Build history of the part. All positions in model axes, mm. A direction names the side the tool comes from. Give positions to 0.01 mm unless a question says otherwise; leave off trailing zeros. Loops run counter-clockwise (first coordinate to the right, second up) from the corner with the lowest first, then second, coordinate; pieces in that order, holes last. Notation, with made-up numbers: (48.25, 15) -> (92.25, 15) arc R24 cw to (92.25, 34) -> close; hole circle Ø2 at (6.5, -1). An arc over 180 degrees is marked (long way). Answer in a Markdown table with one row per item. Add a question column.
from build123d import *

# Parameters (mm, degrees)
SKETCH1_R              = 8
BOSS_EXTRUDE1_DEPTH    = 130
FILLET1_R              = 20
SKETCH2_W              = 2
SKETCH2_H              = 130
BOSS_EXTRUDE4_DEPTH    = 30
CUT_EXTRUDE1_DEPTH     = 9
FILLET2_R              = 1
FILLET3_R              = 2
CUT_EXTRUDE2_START     = -11
CUT_EXTRUDE2_OUTLINE_W = 137
CUT_EXTRUDE2_OUTLINE_H = 54
CUT_EXTRUDE2_DEPTH     = 11
CUT_EXTRUDE3_DEPTH     = 50
SKETCH6_W              = 87.560859394
SKETCH6_H              = 110.580871242
SKETCH6_RX             = 28
SKETCH6_RY             = 6.639736886
SKETCH6_RY_2           = 5.950557319
BOSS_EXTRUDE7_DEPTH    = 1.5
SKETCH7_W              = 87.560859394
SKETCH7_H              = 1.5
CUT_EXTRUDE4_DEPTH     = 0.290435621
SKETCH8_W              = 87.560859394
SKETCH8_H              = 1.5
CUT_EXTRUDE5_DEPTH     = 0.290435621
SKETCH9_R              = 113.429913181
CUT_EXTRUDE6_DEPTH     = 135
SKETCH10_W             = 60.632055489
SKETCH10_H             = 78.176650268
BOSS_EXTRUDE8_DEPTH    = 4.5
SKETCH11_R             = 8.1
CUT_EXTRUDE7_DEPTH     = 135
SKETCH12_W             = 3
SKETCH12_H             = 110
BOSS_EXTRUDE9_DEPTH    = 51
FILLET4_R              = 10
FILLET5_R              = 1.5
FILLET7_R              = 1


# Read off the part's stored shape, not the designer's step: Cut-Extrude2
with BuildPart() as part:
    # Sketch1 → Boss-Extrude1 (new body)
    with BuildSketch(Plane(origin=(0, 0, 0), x_dir=(1, 0, 0), z_dir=(0, 1, 0))):
        with BuildLine():
            ThreePointArc((-62.734857267, 11), (-66.796876469, -10.22252415), (-55.185022832, 8))
            Line((-55.185022832, 8), (41.715308298, 8))
            ThreePointArc((41.715308298, 8), (53.327161935, -10.22252415), (49.265142733, 11))
            Line((49.265142733, 11), (-62.734857267, 11))
        make_face()
        with Locations(Location((-62.734857267, 0, 0), (0, 0, 270))):
            Circle(SKETCH1_R, mode=Mode.SUBTRACT)
        with Locations(Location((49.265142733, 0, 0), (0, 0, 270))):
            Circle(SKETCH1_R, mode=Mode.SUBTRACT)
    extrude(amount=BOSS_EXTRUDE1_DEPTH)

    # Fillet1
    fillet1_edges = [part.edges().sort_by_distance(p)[0] for p in [
        (41.715308298, 65, -8),
        (-55.185022832, 65, -8),
    ]]
    fillet(fillet1_edges, radius=FILLET1_R)

    # Sketch2 → Boss-Extrude4 (add)
    with BuildSketch(Plane(origin=(0, 0, -11), x_dir=(-1, 0, 0), z_dir=(0, 0, -1))):
        with Locations((7.734857267, 65)):
            Rectangle(SKETCH2_W, SKETCH2_H)
        with Locations((5.734857267, 65)):
            Rectangle(SKETCH2_W, SKETCH2_H)
    extrude(amount=BOSS_EXTRUDE4_DEPTH)

    # Sketch3 → Cut-Extrude1 (cut)
    with BuildSketch(Plane(origin=(0, 130, 0), x_dir=(1, 0, 0), z_dir=(0, 1, 0))):
        with BuildLine():
            Line((-34.151645411, 8), (20.681930877, 8))
            ThreePointArc((20.681930877, 8), (31.753545265, 4.655910508), (39.12271272, -4.258064516))
            ThreePointArc((39.12271272, -4.258064516), (58.425893512, -6.089387914), (49.265142733, 11))
            Line((49.265142733, 11), (-4.734857267, 11))
            Line((-4.734857267, 11), (-4.734857267, 41))
            Line((-4.734857267, 41), (-8.734857267, 41))
            Line((-8.734857267, 41), (-8.734857267, 11))
            Line((-8.734857267, 11), (-62.734857267, 11))
            ThreePointArc((-62.734857267, 11), (-71.895608046, -6.089387914), (-52.592427254, -4.258064516))
            ThreePointArc((-52.592427254, -4.258064516), (-45.223259799, 4.655910508), (-34.151645411, 8))
        make_face()
    extrude(amount=-CUT_EXTRUDE1_DEPTH, mode=Mode.SUBTRACT)

    # Fillet2
    fillet2_edges = [part.edges().sort_by_distance(p)[0] for p in [
        (-8.734857267, 60.5, -11),
        (-4.734857267, 60.5, -11),
    ]]
    fillet(fillet2_edges, radius=FILLET2_R)

    # Fillet3
    fillet3_edges = [part.edges().sort_by_distance(p)[0] for p in [
        (-4.734857267, 60.5, -41),
        (-8.734857267, 60.5, -41),
    ]]
    fillet(fillet3_edges, radius=FILLET3_R - 0.0001)  # a hair under: the kernel refuses the full size

    # Cut-Extrude2 outline → Cut-Extrude2 (cut)
    with BuildSketch(Plane.XZ.offset(CUT_EXTRUDE2_START)):
        with Locations((-6.5, -15)):
            Rectangle(CUT_EXTRUDE2_OUTLINE_W, CUT_EXTRUDE2_OUTLINE_H)
    extrude(amount=CUT_EXTRUDE2_DEPTH, mode=Mode.SUBTRACT)

    # Sketch5 → Cut-Extrude3 (cut)
    with BuildSketch(Plane(origin=(0, 0, -11), x_dir=(-1, 0, 0), z_dir=(0, 0, -1))):
        with BuildLine():
            add(Edge.make_bspline(
                [(27.082988225, 66), (27.082988225, 94), (20.443251339, 94)],
                knots=[1.570796327, 1.570796327, 1.570796327, 3.141592654, 3.141592654, 3.141592654], degree=2, weights=[1, 0.707106781, 1]))
            Line((20.443251339, 94), (20.443251339, 66))
            Line((20.443251339, 66), (27.082988225, 66))
        make_face()
        with BuildLine():
            Line((20.443251339, 66), (20.443251339, 94))
            add(Edge.make_bspline(
                [(20.443251339, 94), (13.803514453, 94), (13.803514453, 66)],
                knots=[3.141592654, 3.141592654, 3.141592654, 4.71238898, 4.71238898, 4.71238898], degree=2, weights=[1, 0.707106781, 1]))
            Line((13.803514453, 66), (20.443251339, 66))
        make_face()
        with BuildLine():
            Line((20.443251339, 66), (13.803514453, 66))
            add(Edge.make_bspline(
                [(13.803514453, 66), (13.803514453, 38), (20.443251339, 38)],
                knots=[4.71238898, 4.71238898, 4.71238898, 6.283185307, 6.283185307, 6.283185307], degree=2, weights=[1, 0.707106781, 1]))
            add(Edge.make_bspline(
                [(20.443251339, 38), (27.082988225, 38), (27.082988225, 66)],
                knots=[0, 0, 0, 1.570796327, 1.570796327, 1.570796327], degree=2, weights=[1, 0.707106781, 1]))
            Line((27.082988225, 66), (20.443251339, 66))
        make_face()
        with BuildLine():
            Line((-1.022979486, 66), (-6.973536805, 66))
            Line((-6.973536805, 66), (-12.924094124, 66))
            add(Edge.make_bspline(
                [(-12.924094124, 66), (-12.924094124, 38), (-6.973536805, 38)],
                knots=[4.71238898, 4.71238898, 4.71238898, 6.283185307, 6.283185307, 6.283185307], degree=2, weights=[1, 0.707106781, 1]))
            add(Edge.make_bspline(
                [(-6.973536805, 38), (-1.022979486, 38), (-1.022979486, 66)],
                knots=[0, 0, 0, 1.570796327, 1.570796327, 1.570796327], degree=2, weights=[1, 0.707106781, 1]))
        make_face()
        with BuildLine():
            add(Edge.make_bspline(
                [(-1.022979486, 66), (-1.022979486, 94), (-6.973536805, 94)],
                knots=[1.570796327, 1.570796327, 1.570796327, 3.141592654, 3.141592654, 3.141592654], degree=2, weights=[1, 0.707106781, 1]))
            Line((-6.973536805, 94), (-6.973536805, 66))
            Line((-6.973536805, 66), (-1.022979486, 66))
        make_face()
        with BuildLine():
            Line((-6.973536805, 66), (-6.973536805, 94))
            add(Edge.make_bspline(
                [(-6.973536805, 94), (-12.924094124, 94), (-12.924094124, 66)],
                knots=[3.141592654, 3.141592654, 3.141592654, 4.71238898, 4.71238898, 4.71238898], degree=2, weights=[1, 0.707106781, 1]))
            Line((-12.924094124, 66), (-6.973536805, 66))
        make_face()
    extrude(amount=-CUT_EXTRUDE3_DEPTH, mode=Mode.SUBTRACT)

    # Sketch6 → Boss-Extrude7 (add)
    with BuildSketch(Plane.XY.offset(-8)):
        with Locations((-6.734857267, 66)):
            Rectangle(SKETCH6_W, SKETCH6_H)
        with Locations(Location((-20.443251339, 66), (0, 0, -90))):
            Ellipse(SKETCH6_RX, SKETCH6_RY, mode=Mode.SUBTRACT)
        with Locations(Location((6.973536805, 66), (0, 0, -90))):
            Ellipse(SKETCH6_RX, SKETCH6_RY_2, mode=Mode.SUBTRACT)
    extrude(amount=BOSS_EXTRUDE7_DEPTH)

    # Sketch7 → Cut-Extrude4 (cut)
    with BuildSketch(Plane(origin=(0, 121.290435621, 0), x_dir=(1, 0, 0), z_dir=(0, 1, 0))):
        with Locations((-6.734857267, 7.25)):
            Rectangle(SKETCH7_W, SKETCH7_H)
    extrude(amount=-CUT_EXTRUDE4_DEPTH, mode=Mode.SUBTRACT)

    # Sketch8 → Cut-Extrude5 (cut)
    with BuildSketch(Plane.XZ.offset(-10.709564379)):
        with Locations((-6.734857267, -7.25)):
            Rectangle(SKETCH8_W, SKETCH8_H)
    extrude(amount=-CUT_EXTRUDE5_DEPTH, mode=Mode.SUBTRACT)

    # Sketch9 → Cut-Extrude6 (cut)
    with BuildSketch(Plane(origin=(0, 0, -11), x_dir=(-1, 0, 0), z_dir=(0, 0, -1))):
        with Locations((15.997363152, 101.645153737)):
            Circle(SKETCH9_R)
    extrude(amount=CUT_EXTRUDE6_DEPTH, mode=Mode.SUBTRACT)

    # Sketch10 → Boss-Extrude8 (add)
    with BuildSketch(Plane(origin=(0, 0, -11), x_dir=(-1, 0, 0), z_dir=(0, 0, -1))):
        with Locations((5.573817907, 65.992517727)):
            Rectangle(SKETCH10_W, SKETCH10_H)
    extrude(amount=-BOSS_EXTRUDE8_DEPTH)

    # Sketch11 → Cut-Extrude7 (cut)
    with BuildSketch(Plane.XZ.offset(-11)):
        with Locations(Location((-62.734857267, 0, 0), (0, 0, 270))):
            Circle(SKETCH11_R)
        with Locations(Location((49.265142733, 0, 0), (0, 0, 270))):
            Circle(SKETCH11_R)
    extrude(amount=-CUT_EXTRUDE7_DEPTH, mode=Mode.SUBTRACT)

    # Sketch12 → Boss-Extrude9 (add)
    with BuildSketch(Plane(origin=(0, 0, -11), x_dir=(-1, 0, 0), z_dir=(0, 0, -1))):
        with Locations((-22.265142733, 66)):
            Rectangle(SKETCH12_W, SKETCH12_H)
        with Locations((35.734857267, 66)):
            Rectangle(SKETCH12_W, SKETCH12_H)
    extrude(amount=BOSS_EXTRUDE9_DEPTH)

    # Fillet4
    fillet4_edges = [part.edges().sort_by_distance(p)[0] for p in [
        (23.765142733, 66, -11),
        (-37.234857267, 66, -11),
    ]]
    fillet(fillet4_edges, radius=FILLET4_R)

    # Fillet5
    fillet5_edges = [part.edges().sort_by_distance(p)[0] for p in [
        (20.765142733, 66, -11),
        (-34.234857267, 66, -11),
    ]]
    fillet(fillet5_edges, radius=FILLET5_R)

    # Fillet7
    fillet7_edges = [part.edges().sort_by_distance(p)[0] for p in [
        (23.765142733, 66, -62),
        (22.265142733, 11, -62),
        (20.765142733, 66, -62),
        (22.265142733, 121, -62),
        (-37.234857267, 66, -62),
        (-35.734857267, 121, -62),
        (-34.234857267, 66, -62),
        (-35.734857267, 11, -62),
    ]]
    fillet(fillet7_edges, radius=FILLET7_R)


solid = part.part
(1) Saw through at C-C, the plane z = 0. List the corners of the cut face in (x, y), then the cut area to 3 significant figures.
(2) Saw through at B-B, the plane y = 27. List the corners of the cut face in (x, z).
(3) Saw through at A-A, the plane z = -37. List the corners of the cut face in (x, y), then the cut area to 3 significant figures.
(4) Saw through at D-D, the plane x = -23. List the corners of the cut face in (y, z), then the cut area to 3 significant figures.
(5) Two-plate mould, pull along X, no slides. Class faces 1 (the cylindrical face through (-40.242, 66.77, -13.852)), 2 (the flat face through (-55, 65, -11)), 3 (the cylindrical face through (-55.9, 65.23, -4.35)): released by +X, released by -X, zero draft, split by the parting line, or undercut.
(6) Flat gauge pins, fed straight in: pin 1 Ø12 at (y, z) = (26, -29) entering from -X; pin 2 Ø3 at (x, y) = (-34.5, 97.5) entering from +Z; pin 3 Ø4 at (x, y) = (-23.5, 56) entering from -Z; pin 4 Ø9.5 at (x, z) = (-62.73, 0) entering from -Y. Where does each tip first touch, or does it go through?
(7) 3-axis set-ups, long thin cutter, end or side, ignore diameter. For faces 4 (the flat face through (-7, 67, -6.5)), 5 (the cylindrical face through (58.24, 65.23, 6.36)), 6 (the flat face through (23.765, 65, -41)), 7 (the flat face through (-37.235, 65, -41)), 8 (the flat face through (-6, 65, -11)): which of +Z, -Z, +X, -X, +Y, -Y reach the whole face in a straight line?
(8) Wall check: line 1 along X through (y, z) = (24, -34); line 2 along X through (y, z) = (64, 0); line 3 along X through (y, z) = (21, 2). Give the ranges that are in metal, low to high. Write a range as from..to.
Worked answers:
| question | item | result |
|---|---|---|
| 1 | outline | (-73.73, 11) -> (-70.83, 11) -> (-70.83, 121) -> (-73.73, 121) -> close; (-54.63, 11) -> (-50.15, 11) -> (-50.15, 121) -> (-54.63, 121) -> close; (36.68, 11) -> (41.17, 11) -> (41.17, 121) -> (36.68, 121) -> close; (57.37, 11) -> (60.27, 11) -> (60.27, 121) -> (57.37, 121) -> close |
| 1 | area | 1,620 mm^2 |
| 2 | outline | (-62.73, -11) -> (-47.23, -11) arc R10 cw to (-37.23, -21) -> (-37.23, -61) arc R1 ccw to (-36.23, -62) -> (-35.23, -62) arc R1 ccw to (-34.23, -61) -> (-34.23, -12.5) arc R1.5 cw to (-32.73, -11) -> (19.27, -11) arc R1.5 cw to (20.77, -12.5) -> (20.77, -61) arc R1 ccw to (21.77, -62) -> (22.77, -62) arc R1 ccw to (23.77, -61) -> (23.77, -21) arc R10 cw to (33.77, -11) -> (49.27, -11) arc R11 ccw (long way) to (39.12, 4.26) arc R20 cw to (28.28, -6.5) -> (-41.75, -6.5) arc R20 cw to (-52.59, 4.26) arc R11 ccw (long way) to start; hole circle Ø16.2 at (-62.73, 0); hole circle Ø16.2 at (49.27, 0) |
| 3 | outline | (-37.23, 11) -> (-34.23, 11) -> (-34.23, 121) -> (-37.23, 121) -> close; (20.77, 11) -> (23.77, 11) -> (23.77, 121) -> (20.77, 121) -> close |
| 3 | area | 660 mm^2 |
| 4 | outline | (11, -11) -> (121, -11) -> (121, -6.5) -> (11, -6.5) -> close |
| 4 | area | 495 mm^2 |
| 5 | face 1 | released by -X |
| 5 | face 2 | zero draft |
| 5 | face 3 | undercut |
| 6 | pin 1 | x = -37.23 |
| 6 | pin 2 | z = -6.5 |
| 6 | pin 3 | z = -11 |
| 6 | pin 4 | through |
| 7 | face 4 | +Z, +Y, -Y |
| 7 | face 5 | +Y, -Y |
| 7 | face 6 | -Z, +X, +Y, -Y |
| 7 | face 7 | -Z, -X, +Y, -Y |
| 7 | face 8 | -Z, +Y, -Y |
| 8 | line 1 | -37.23..-34.23, 20.77..23.77 |
| 8 | line 2 | -73.73..-70.83, -54.63..-50.15, 36.68..41.17, 57.37..60.27 |
| 8 | line 3 | -73.55..-70.58, -54.89..-51.47, 38..41.42, 57.11..60.08 |
